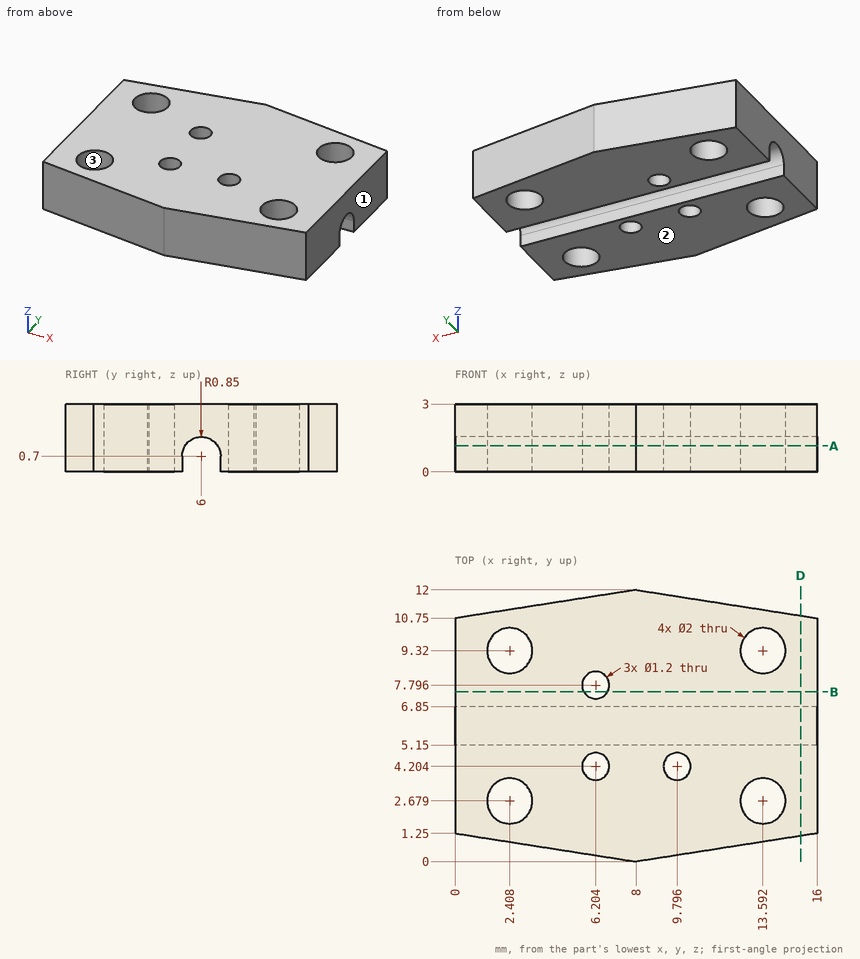
Check sheet for the drawn part. Datum: minimum x, y, z corner. Units: mm. Give positions to 0.01 mm unless a question says otherwise; leave off trailing zeros. Write each loop counter-clockwise with the first axis right and the second up, starting at its lowest first coordinate (ties: lowest second). Pieces come first, ordered by that corner, then holes. Notation, with made-up numbers: (-25, 27) -> (-17, 27) arc R28 cw to (-17, 66) -> close; hole circle Ø4 at (76.25, -39). An arc over 180 degrees is marked (long way). Use one line per item in the form item = value. Start each with the question number.
1. Thickness scan on line 1 along X through (y, z) = (3.75, 2.4) (1 decimal); line 2 along X through (y, z) = (2.75, 1.75) (1 decimal); line 3 along Y through (x, z) = (2.75, 0.6). Record the ranges inside material, lowest first. Write a range as from..to.
2. Mould release check, pull along X, two halves, no side actions. Record for the marked faces 1, 2 and 3: pulls with the +X half, pulls with the -X half, needs draft (parallel to the pull), parting line crosses it, or undercut.
3. Go/stop test with flat-tipped pins: P1, Ø1.6, axis at x = 13.59, y = 2.68, coming from the +Z side; P2, Ø0.6, axis at x = 4.5, z = 0.5, coming from the -Y side. Record where each tip stops, or that it passes through.
4. Section check D-D (x = 15.25). Record the cut outline in (y, z), and give its area (3 significant figures).
5. Section check A-A (z = 1.15). Count the separate pieces of the cut face and the enclosed holes in it, and give its area (3 significant figures).
6. Section check B-B (y = 7.5). Record the cut outline in (x, z) (1 decimal).
Conclusion:
q1.line_1 = 0..5.8, 6.6..9.4, 10.2..16
q1.line_2 = 0..1.4, 3.4..12.6, 14.6..16
q1.line_3 = 0.82..1.74, 3.62..5.15, 6.85..8.38, 10.26..11.18
q2.face_1 = pulls with the +X half
q2.face_2 = needs draft
q2.face_3 = undercut
q3.P1 = through
q3.P2 = 0.5
q4.outline = (1.13, 0) -> (5.15, 0) -> (5.15, 0.7) arc R0.85 cw to (6.85, 0.7) -> (6.85, 0) -> (10.87, 0) -> (10.87, 3) -> (1.13, 3) -> close
q4.area = 26.9 mm²
q5.separate_pieces = 2
q5.enclosed_holes = 7
q5.area = 133 mm²
q6.outline = (0, 0) -> (5.7, 0) -> (5.7, 3) -> (0, 3) -> close; (6.7, 0) -> (16, 0) -> (16, 3) -> (6.7, 3) -> close
